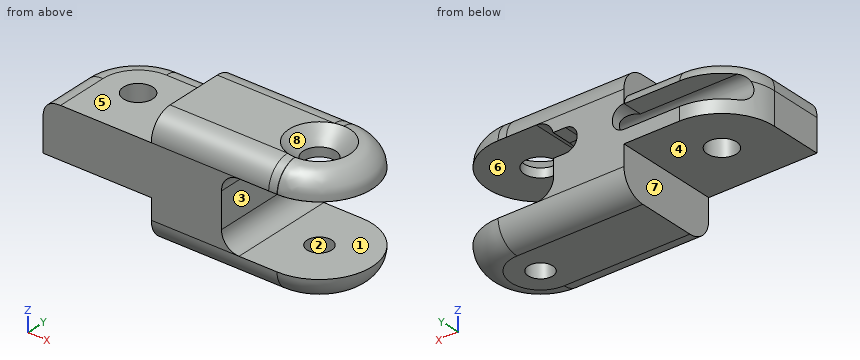
from build123d import *

# Parameters (mm, degrees)
BOSS_EXTRUDE1_DEPTH         = 18
SKETCH5_OUTSIDE_W           = 62.18
SKETCH5_OUTSIDE_H           = 31.18
SKETCH5_OUTSIDE_R           = 2.5
CUT_EXTRUDE1_DEPTH          = 20
M5_TAPPED_HOLE1_D           = 4.2
M5_TAPPED_HOLE1_CSINK_D     = 10.4
M5_TAPPED_HOLE1_CSINK_ANGLE = 90
FILLET1_R                   = 4
FILLET2_R                   = 4
FILLET3_SIZE                = 3
CUT_EXTRUDE2_DEPTH          = 37.800136028
CUT_EXTRUDE2_DEPTH_BACK     = 37.800136028
SKETCH12_R                  = 2
CUT_EXTRUDE3_DEPTH          = 3.5
CUT_EXTRUDE4_DEPTH          = 3.5


# Some blends are built 0.0001 mm under size
with BuildPart() as part:
    # Sketch2 → Boss-Extrude1 (new body)
    with BuildSketch(Plane(origin=(0, 0, 0), x_dir=(1, 0, 0), z_dir=(0, 1, 0))):
        with BuildLine():
            Line((-6, 10), (24.5, 10))
            Line((24.5, 10), (24.5, 6))
            Line((24.5, 6), (9, 6))
            ThreePointArc((9, 6), (6.878679656, 5.121320344), (6, 3))
            Line((6, 3), (6, -3))
            ThreePointArc((6, -3), (6.878679656, -5.121320344), (9, -6))
            Line((9, -6), (24.5, -6))
            Line((24.5, -6), (24.5, -10))
            Line((24.5, -10), (-6, -10))
            Line((-6, -10), (-6, -6))
            Line((-6, -6), (-24.5, -6))
            Line((-24.5, -6), (-24.5, 2.5))
            Line((-24.5, 2.5), (-6, 2.5))
            Line((-6, 2.5), (-6, 10))
        make_face()
    extrude(amount=BOSS_EXTRUDE1_DEPTH)

    # Sketch5 outside → Cut-Extrude1 (cut)
    # profile 1 of 2: a face of its own
    with BuildSketch(Plane.XY.offset(10)):
        with Locations((0, 9)):
            Rectangle(SKETCH5_OUTSIDE_W, SKETCH5_OUTSIDE_H)
        with BuildLine():
            Line((-24.5, 9), (-24.5, 0))
            Line((-24.5, 0), (15.5, 0))
            ThreePointArc((15.5, 0), (24.5, 9), (15.5, 18))
            Line((15.5, 18), (-15.5, 18))
            ThreePointArc((-15.5, 18), (-21.863961031, 15.363961031), (-24.5, 9))
        make_face(mode=Mode.SUBTRACT)
    # profile 2 of 2: a face of its own
    with BuildSketch(Plane.XY.offset(10)):
        with Locations((-15.5, 9)):
            Circle(SKETCH5_OUTSIDE_R)
    extrude(amount=-CUT_EXTRUDE1_DEPTH, mode=Mode.SUBTRACT)

    # Sketch8 → CSK for M5 Countersunk Flat Head Screw1 (revolve, cut)
    with BuildSketch(Plane(origin=(15.5, 9, 10), x_dir=(0, -1, 0), z_dir=(1, 0, 0))):
        Polygon((0, 0), (0, 4), (2.75, 4), (2.75, 2.45), (5.2, 0), align=None)
    revolve(axis=Axis((15.5, 9, 16.35), (0, 0, -1)), mode=Mode.SUBTRACT)

    # M5 Tapped Hole1 (through all)
    with Locations(Plane.XY.offset(10)):
        with Locations((15.5, 9)):
            CounterSinkHole(M5_TAPPED_HOLE1_D / 2, M5_TAPPED_HOLE1_CSINK_D / 2, counter_sink_angle=M5_TAPPED_HOLE1_CSINK_ANGLE)

    # Fillet1
    fillet1_edges = [part.edges().sort_by_distance(p)[0] for p in [
        (4.75, 0, 10),
        (4.75, 18, 10),
    ]]
    fillet(fillet1_edges, radius=FILLET1_R - 0.0001)  # a hair under: the kernel refuses the full size

    # Fillet2
    fillet2_edges = [part.edges().sort_by_distance(p)[0] for p in [
        (4.75, 0, -10),
        (24.5, 9, -10),
        (4.75, 18, -10),
    ]]
    fillet(fillet2_edges, radius=FILLET2_R - 0.0001)  # a hair under: the kernel refuses the full size

    # Fillet3
    # a fillet whose section is not a circle: 3 mm, written as the material it takes off along each edge
    with BuildSketch(Plane(origin=(-24.5, -7.5, 6), x_dir=(0, 0, -1), z_dir=(0, 1, 0))) as fillet3_piece_1:
        with BuildLine():
            Bezier((FILLET3_SIZE, 0), (0, 0), (0, -FILLET3_SIZE), weights=[1, 1, 1])
            Line((0, -FILLET3_SIZE), (0, 0))
            Line((0, 0), (FILLET3_SIZE, 0))
        make_face()
    extrude(amount=16.5, mode=Mode.SUBTRACT)
    with BuildSketch(Plane(origin=(-6, 18, 6), x_dir=(0, -1, 0), z_dir=(-1, 0, 0))) as fillet3_piece_2:
        with BuildLine():
            Bezier((FILLET3_SIZE, 0), (0, 0), (0, -FILLET3_SIZE), weights=[1, 1, 1])
            Line((0, -FILLET3_SIZE), (0, 0))
            Line((0, 0), (FILLET3_SIZE, 0))
        make_face()
    extrude(amount=9.5, mode=Mode.SUBTRACT)
    with BuildSketch(Plane(origin=(-15.5, 9, 6), x_dir=(0, 1, 0), z_dir=(1, 0, 0))) as fillet3_piece_3:
        with BuildLine():
            Bezier((9 - FILLET3_SIZE, 0), (9, 0), (9, -FILLET3_SIZE), weights=[1, 1, 1])
            Line((9, -FILLET3_SIZE), (9, 0))
            Line((9, 0), (9 - FILLET3_SIZE, 0))
        make_face()
    revolve(axis=Axis((-15.5, 9, 6), (0, 0, 1)), revolution_arc=90, mode=Mode.SUBTRACT)

    # Sketch12 → Cut-Extrude2 (cut, two sides: drawn at the far end of the back side and taken through both)
    with BuildSketch(Plane(origin=(6, 0, 0), x_dir=(0, 0, -1), z_dir=(1, 0, 0)).offset(-CUT_EXTRUDE2_DEPTH_BACK)):
        with Locations(Location((-1.75, 14.5, 0), (0, 0, 231.317812547))):
            Circle(SKETCH12_R)
    extrude(amount=CUT_EXTRUDE2_DEPTH + CUT_EXTRUDE2_DEPTH_BACK, mode=Mode.SUBTRACT)

    # Sketch13 → Cut-Extrude3 (cut)
    with BuildSketch(Plane(origin=(0, 18, 0), x_dir=(1, 0, 0), z_dir=(0, 1, 0))):
        with BuildLine():
            Line((-24, 0.25), (-6, 0.25))
            ThreePointArc((-6, 0.25), (-4, -1.75), (-6, -3.75))
            Line((-6, -3.75), (-24, -3.75))
            Line((-24, -3.75), (-24, 0.25))
        make_face()
    extrude(amount=-CUT_EXTRUDE3_DEPTH, mode=Mode.SUBTRACT)

    # Sketch15 → Cut-Extrude4 (cut)
    with BuildSketch(Plane(origin=(0, 18, 0), x_dir=(1, 0, 0), z_dir=(0, 1, 0))):
        with BuildLine():
            Line((4, 0.25), (9, 0.25))
            Line((9, 0.25), (9, -3.75))
            Line((9, -3.75), (4, -3.75))
            ThreePointArc((4, -3.75), (2, -1.75), (4, 0.25))
        make_face()
    extrude(amount=-CUT_EXTRUDE4_DEPTH, mode=Mode.SUBTRACT)


solid = part.part
The model under review builds one solid part; all positions refer to its coordinate system, in mm. Face numbers are marked on the shaded views. A direction names the side the tool comes from. Round coordinates to 2 decimals unless told otherwise and drop trailing zeros. Loops run counter-clockwise (first coordinate to the right, second up) from the corner with the lowest first, then second, coordinate; pieces in that order, holes last. Notation, with made-up numbers: (77.25, -28) -> (120.25, -28) arc R12 cw to (120.25, -10) -> close; hole circle Ø3 at (25, 56.5). An arc over 180 degrees is marked (long way). One line per question, with ' | ' between items. Start each with the question number.
Item 1: Machinability: for the marked faces 5, 6, 7 and 8, which of the approach directions +Z, -Z, +X, -X, +Y, -Y give a long, thin tool a straight path to every point of the face, cutting with its end or side? Answer none if there is none.
Item 2: Add section A-A, the plane z = -4.5. Write out the cut boundary in (x, y).
Item 3: Draft analysis for pull direction Z (two halves, no side actions). For the marked faces 1, 2, 3 and 4, state which applies: +Z half, -Z half, draft (parallel to the pull), parting line (faces both ways), or undercut.
Item 4: For pin 1 (7 mm diameter, centred on y = 9, z = 7, fed in from -X); pin 2 (9 mm diameter, centred on x = -14.5, y = 12, fed in from -Z); pin 3 (1.8 mm diameter, centred on x = -17, y = 15.5, fed in from +Z), all flat-tipped, find the tip position at first contact; note any pin that passes through.
Item 5: Wall thickness on line 1 along X through (y, z) = (2, 1.25); line 2 along Z through (x, y) = (-15, 14.5); line 3 along Z through (x, y) = (-13, 3.75): over which ranges is each line inside the solid? List them lowest first. Write a range as [from, to].
Return value:
1) face 5: +Z, -X, +Y, -Y | face 6: +X, +Y, -Y | face 7: -Z, -X, +Y, -Y | face 8: +Z
2) outline: (-6, 0) -> (6.4, 0) -> (6.4, 18) -> (-6, 18) -> close
3) face 1: undercut | face 2: draft | face 3: undercut | face 4: -Z half
4) pin 1: stops at x = -24.48 | pin 2: stops at z = -2.5 | pin 3: stops at z = 6
5) line 1: x = [-24.5, 6] | line 2: z = [-2.5, -0.25], [3.75, 6] | line 3: z = [-2.5, 6]
